For this review, take the finished solid that the model builds, in its own axes (mm). Coordinates: 2 decimals unless noted, no trailing zeros. Order: outer loops, then holes, each group sorted by start corner. A loop starts at its lowest first (then second) coordinate and runs counter-clockwise, first axis right, second up. Notation, with made-up numbers: (-22, 20.5) - (-11, 20.5) arc R21 cw to (-11, 37.5) - close; hole circle Ø10 at (81, 61). An arc over 180 degrees is marked (long way). One line per item, written item: value. Start each with the question number.
(1) Mouldability with a two-part tool opening along Y and no side actions: class faces 1 (the cylindrical face through (-27.68, -24.05, 0.78)), 2 (the cylindrical face through (-30.44, -4.37, 0.78)), 3 (the flat face through (-21, -11, 1.588)), 4 (the flat face through (-15.22, -4.11, 0.78)) as released by +Y, released by -Y, zero draft, split by the parting line, or undercut.
(2) Consider section B-B on z = 0.75. Write out the cut boundary in (x, y).
(3) Consider section D-D on x = -25.5. Write out the cut boundary in (y, z), then the cut area to 3 significant figures.
(4) Consider section C-C on y = -22. Write out the cut boundary in (x, z), then the cut area to 3 significant figures.
(5) To check wall thickness, follow line 1 along Y through (x, z) = (-4, 0.85); line 2 along X through (y, z) = (-3, 1.05); line 3 along Y through (x, z) = (-33, 0.65). State the ranges of each line that lie inside material, in increasing order.
(6) Consider section A-A on x = -31.5. Write out the cut boundary in (y, z).
Autodesk Inventor part; units mm, degrees
ref_plane "YZ Plane" through (0, 0, 0) normal (1, 0, 0) x (0, 1, 0)
ref_plane "XZ Plane" through (0, 0, 0) normal (0, 1, 0) x (-1, 0, 0)
ref_plane "XY Plane" through (0, 0, 0) normal (0, 0, 1) x (1, 0, 0)
sketch "Sketch1" plane through (0, 0, 0) normal (0, 0, 1) x (1, 0, 0)
  circle A0 centre (-5.4749, -29.1324) radius 2.1844
  line L0 (-37.2249, 22.5069) -> (-37.2249, -1.3553)
  arc A1 (-35.2179, 22.7309) -> (-37.2249, 22.5069) centre (-36.2089, 22.5069) ccw
  line L1 (3.1159, -33.1053) -> (-5.4749, -33.1053)
  arc A2 (3.1159, -33.1053) -> (4.3913, -30.5726) centre (3.1159, -31.5178) ccw
  arc A3 (-37.2249, -1.3553) -> (-5.4749, -33.1053) centre (-5.4749, -1.3553) ccw
  circle A4 centre (-32.4624, -3.7324) radius 2.1209
  line L2 (4.3913, -30.5726) -> (-35.3926, 23.1119)
  point P0 (0, 0)
  point P1 (-37.2249, 40.7176)
  point P2 (9.6063, -33.1053)
  dimension "d0" = 1.016
  dimension "d1" = 1.5875
  dimension "d2" = 31.75
extrude "Extrusion1" add sketch "Sketch1" along normal blind 1.5875
properties part number "ramp_v2"
Geometry check:
1. face 1: released by -Y
1. face 2: undercut
1. face 3: zero draft
1. face 4: released by +Y
2. outline: (-37.22, -1.36) arc R31.75 ccw to (-5.47, -33.11) - (3.12, -33.11) arc R1.59 ccw to (4.39, -30.57) - (-35.39, 23.11) arc R1.02 ccw to (-37.22, 22.51) - close; hole circle Ø4.24 at (-32.46, -3.73); hole circle Ø4.37 at (-5.47, -29.13)
3. outline: (-25.99, 0) - (9.76, 0) - (9.76, 1.59) - (-25.99, 1.59) - close
3. area: 56.8 mm^2
4. outline: (-29.6, 0) - (-1.96, 0) - (-1.96, 1.59) - (-29.6, 1.59) - close
4. area: 43.9 mm^2
5. line 1: y = -33.11 to -30.74, -27.52 to -19.25
5. line 2: x = -37.18 to -34.45, -30.47 to -16.04
5. line 3: y = -17.18 to -5.78, -1.68 to 19.88
6. outline: (-19.54, 0) - (-5.62, 0) - (-5.62, 1.59) - (-19.54, 1.59) - close; (-1.84, 0) - (17.86, 0) - (17.86, 1.59) - (-1.84, 1.59) - close
